from build123d import *

# Parameters (mm, degrees)
F0_W     = 76.2
F0_H     = 101.6
F0_W_2   = 25.4
F0_H_2   = 30.48
F1_DEPTH = 25.4
F2_W     = 76.462764
F2_H     = 101.884663
F3_DEPTH = 6.35


with BuildPart() as f1:
    # F0 (on Front) → F1 (new body)
    with BuildSketch(Plane.XZ):
        Rectangle(F0_W, F0_H)
        with Locations((-15.480864, -24.765002)):
            Rectangle(F0_W_2, F0_H_2, mode=Mode.SUBTRACT)
        with Locations((16.269136, -24.751032)):
            Rectangle(F0_W_2, F0_H_2, mode=Mode.SUBTRACT)
        with Locations((-15.480864, 18.414998)):
            Rectangle(F0_W_2, F0_H_2, mode=Mode.SUBTRACT)
        with Locations((16.269136, 18.414998)):
            Rectangle(F0_W_2, F0_H_2, mode=Mode.SUBTRACT)
    extrude(amount=-F1_DEPTH)

    # F2 (on Front) → F3 (join)
    with BuildSketch(Plane.XZ):
        with Locations((-2e-06, 0.098533)):
            Rectangle(F2_W, F2_H)
    extrude(amount=F3_DEPTH)


solid = f1.part
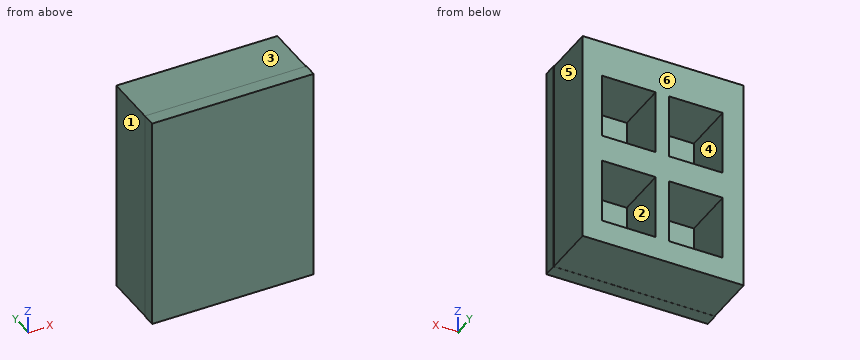
Model file for the job. Use its own axes, mm. Face numbers are marked on the shaded views. A direction names the side the tool comes from. Round coordinates to 2 decimals unless told otherwise and drop trailing zeros. Loops run counter-clockwise (first coordinate to the right, second up) from the corner with the lowest first, then second, coordinate; pieces in that order, holes last. Notation, with made-up numbers: (40, 2.25) -> (67, 2.25) arc R27 cw to (67, 27.25) -> close; hole circle Ø9 at (17, 1). An arc over 180 degrees is marked (long way). Answer as CSV lines item,"result". Start each with the question number.
1) Mould opens along X. For the marked faces 1, 2 and 3 say: +X half, -X half, draft (parallel to the pull), parting line (faces both ways), or undercut.
2) Slice it at B-B (x = 23.5). List the corners of the cut face in (y, z) (3 decimals), plus the area to 3 significant figures.
3) Slice it at A-A (y = 4). List the corners of the cut face in (x, z) (3 decimals).
4) Tool access for the marked faces 4, 5 and 6: list every direction of +Z, -Z, +X, -X, +Y, -Y with a clear straight run to the whole face (end or side of a thin tool).
5) Probe line 1 along X through (y, z) = (5, -11); line 2 along Z through (x, y) = (-27, 22) (3 decimals); line 3 along X through (y, z) = (7, 42). List the from-to ranges inside material, lowest first.
6) Slice it at C-C (z = -28.5). List the corners of the cut face in (x, y), plus the area to 3 significant figures.
7) Pin check, flat tips, straight feed: P1, Ø4, axis at y = 8, z = 28.5, coming from the -X side; P2, Ø10, axis at x = 3.5, y = 20.5, coming from the +Z side; P3, Ø20.5, axis at x = 18, z = 24.5, coming from the +Y side; P4, Ø7.5, axis at y = 8, z = -29, coming from the +X side. Stop position of each tip, or through.
Filled in:
1,face 1,"-X half"
1,face 2,"undercut"
1,face 3,"draft"
2,outline,"(-6.35, -50.844) -> (0, -50.844) -> (0, -50.8) -> (25.4, -50.8) -> (25.4, -39.991) -> (0, -39.991) -> (0, -9.511) -> (25.4, -9.511) -> (25.4, 3.175) -> (0, 3.175) -> (0, 33.655) -> (25.4, 33.655) -> (25.4, 50.8) -> (0, 50.8) -> (0, 51.041) -> (-6.35, 51.041) -> close"
2,area,"1,680 mm2"
3,outline,"(-38.1, -50.8) -> (38.1, -50.8) -> (38.1, 50.8) -> (-38.1, 50.8) -> close; hole (-28.181, -40.005) -> (-2.781, -40.005) -> (-2.781, -9.525) -> (-28.181, -9.525) -> close; hole (-28.181, 3.175) -> (-2.781, 3.175) -> (-2.781, 33.655) -> (-28.181, 33.655) -> close; hole (3.569, -39.991) -> (28.969, -39.991) -> (28.969, -9.511) -> (3.569, -9.511) -> close; hole (3.569, 3.175) -> (28.969, 3.175) -> (28.969, 33.655) -> (3.569, 33.655) -> close"
4,face 4,"+Y"
4,face 5,"+Z, -Z, +X, +Y"
4,face 6,"+Z, -Z, +X, -X, +Y"
5,line 1,"x = -38.1 to -28.18, -2.78 to 3.57, 28.97 to 38.1"
5,line 2,"z = -50.8 to -40.005, -9.525 to 3.175, 33.655 to 50.8"
5,line 3,"x = -38.1 to 38.1"
6,outline,"(-38.23, -6.35) -> (38.23, -6.35) -> (38.23, 0) -> (38.1, 0) -> (38.1, 25.4) -> (28.97, 25.4) -> (28.97, 0) -> (3.57, 0) -> (3.57, 25.4) -> (-2.78, 25.4) -> (-2.78, 0) -> (-28.18, 0) -> (-28.18, 25.4) -> (-38.1, 25.4) -> (-38.1, 0) -> (-38.23, 0) -> close"
6,area,"1,130 mm2"
7,P1,"stops at x = -38.1"
7,P2,"stops at z = 50.8"
7,P3,"stops at y = 25.4"
7,P4,"stops at x = 38.1"
